Study the drawing (mm; zero at the part's minimum x, y, z) and answer. A direction names the side the tool comes from. Give positions to 0.01 mm unless a question says otherwise; leave off trailing zeros. Order: outer loops, then holes, each group sorted by start corner. A loop starts at its lowest first (then second) coordinate and runs counter-clockwise, first axis right, second up. Notation, with made-up numbers: (51.5, -38) - (78.5, -38) arc R20 ccw to (78.5, -16) - close; hole circle Ø1 at (15.25, 21.5). An arc over 180 degrees is marked (long way). Use CSV: the item, a comma, the result in double quotes.
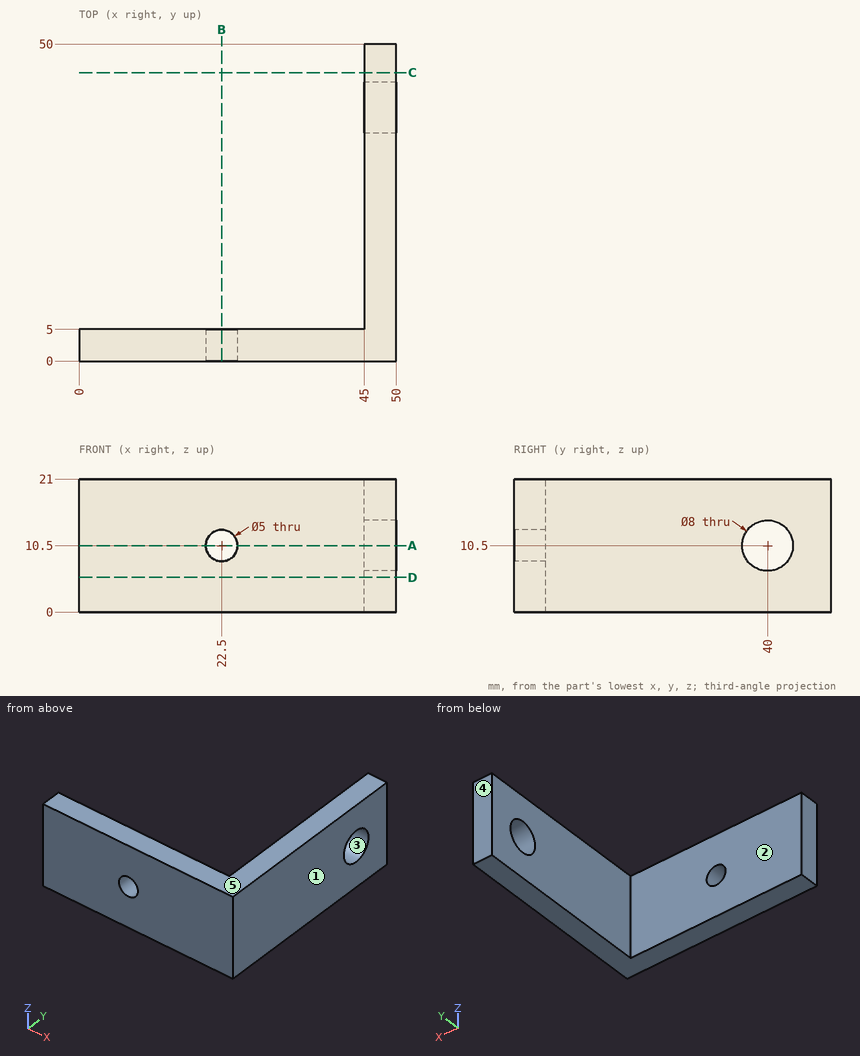
Item 1: The part is cut by section B-B (x = 22.5). Give the vertices of the cut face in (y, z), and give its area (3 significant figures).
Taken from the geometry:
outline,"(0, 0) - (5, 0) - (5, 8) - (0, 8) - close; (0, 13) - (5, 13) - (5, 21) - (0, 21) - close"
area,"80.0 mm^2"
Item 2: Each of these flat-tipped pins is pushed along its axis until it touches: pin 1 (1 mm diameter, centred on y = 19.5, z = 18, fed in from -X); pin 2 (9 mm diameter, centred on y = 40, z = 10.5, fed in from +X); pin 3 (10 mm diameter, centred on x = 23, z = 10, fed in from +Y). Where does it stop, or does it pass through?
Taken from the geometry:
pin 1,"x = 45"
pin 2,"x = 50"
pin 3,"y = 5"
Item 3: The mould has two halves that part along Z. Classify the marked faces 3, 4 and 5: +Z half, -Z half, draft (parallel to the pull), parting line (faces both ways), or undercut.
Taken from the geometry:
face 3,"undercut"
face 4,"draft"
face 5,"+Z half"
Item 4: The part is cut by section A-A (z = 10.5). Give the vertices of the cut face in (x, y).
Taken from the geometry:
outline,"(0, 0) - (20, 0) - (20, 5) - (0, 5) - close; (25, 0) - (50, 0) - (50, 36) - (45, 36) - (45, 5) - (25, 5) - close; (45, 44) - (50, 44) - (50, 50) - (45, 50) - close"
Item 5: Find the intervals of material crossed by line 1 along Z through (x, y) = (46.2, 40); line 2 along X through (y, z) = (2.35, 10.5); line 3 along Z through (x, y) = (22.5, 3.45), in increasing order.
Taken from the geometry:
line 1,"0 to 6.5, 14.5 to 21"
line 2,"0 to 20, 25 to 50"
line 3,"0 to 8, 13 to 21"
Item 6: Which of the six approach directions +Z, -Z, +X, -X, +Y, -Y give full straight-line access (tool end or side, diameter ignored) to the marked faces 1 and 2?
Taken from the geometry:
face 1,"+Z, -Z, +X, +Y, -Y"
face 2,"+Z, -Z, -X, +Y"
Item 7: The part is cut by section D-D (z = 5.5). Give the vertices of the cut face in (x, y), and give its area (3 significant figures).
Taken from the geometry:
outline,"(0, 0) - (50, 0) - (50, 50) - (45, 50) - (45, 5) - (0, 5) - close"
area,"475 mm^2"
Item 8: The part is cut by section C-C (y = 45.5). Give the vertices of the cut face in (x, z).
Taken from the geometry:
outline,"(45, 0) - (50, 0) - (50, 21) - (45, 21) - close"
